Input: dimensioned drawing with shaded views. Units: mm. Origin: part minimum x, y, z. A direction names the side the tool comes from. Coordinates: 2 decimals unless noted, no trailing zeros. One line per question, with ' | ' between items. Start each with the question number.
(1) Draft query along Y for the marked faces 3, 4, 5 and 6. Return one class per face: +Y half, -Y half, draft (parallel to the pull), parting line (faces both ways), or undercut.
(2) Line query: line 1 along Y through (x, z) = (7.75, 1.25); line 2 along Y through (x, z) = (3.5, 11.25); line 3 along Y through (x, z) = (6.25, 9.75). Output: solid intervals per line, ascending.
(3) Section A-A (z = 4). Count the separate pieces of the cut face and the enclosed holes in it, then the cut area to 3 significant figures.
(4) Access query for the marked faces 1 and 2. Directions: +Z, -Z, +X, -X, +Y, -Y. A direction counts if a zero-diameter tool reaches every point of the face in a straight line with its end or side. Return the directions, or none.
(5) Contact query for a flat-ended pin moving along its axis: P1, Ø4.5, axis at x = 4.76, y = 40.55, coming from the +Z side. Output: stop coordinate, or through.
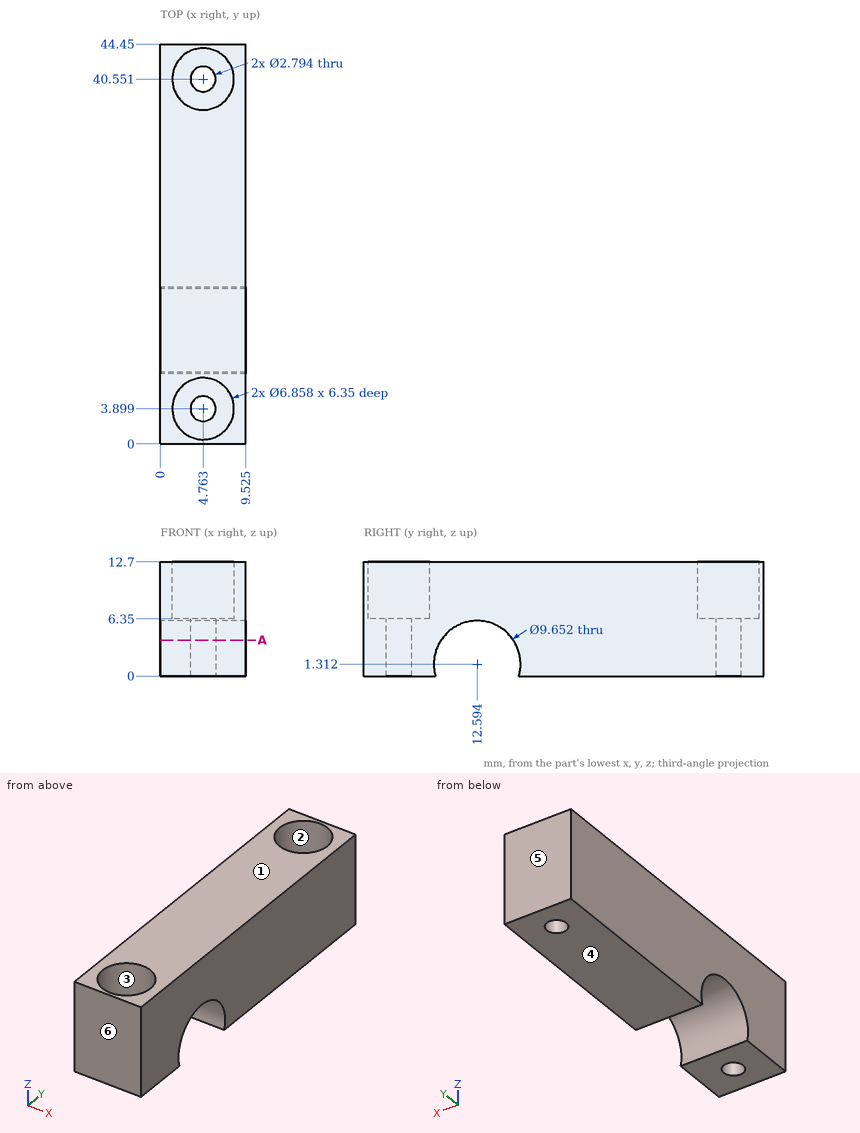
Response values:
1) face 3: undercut | face 4: draft | face 5: +Y half | face 6: -Y half
2) line 1: y = 0 to 7.77, 17.42 to 44.45 | line 2: y = 0 to 0.71, 7.09 to 37.36, 43.74 to 44.45 | line 3: y = 0 to 0.81, 6.99 to 37.46, 43.64 to 44.45
3) separate pieces: 2 | enclosed holes: 2 | area: 335 mm²
4) face 1: +Z, +X, -X, +Y, -Y | face 2: +Z
5) P1: stops at z = 6.35
